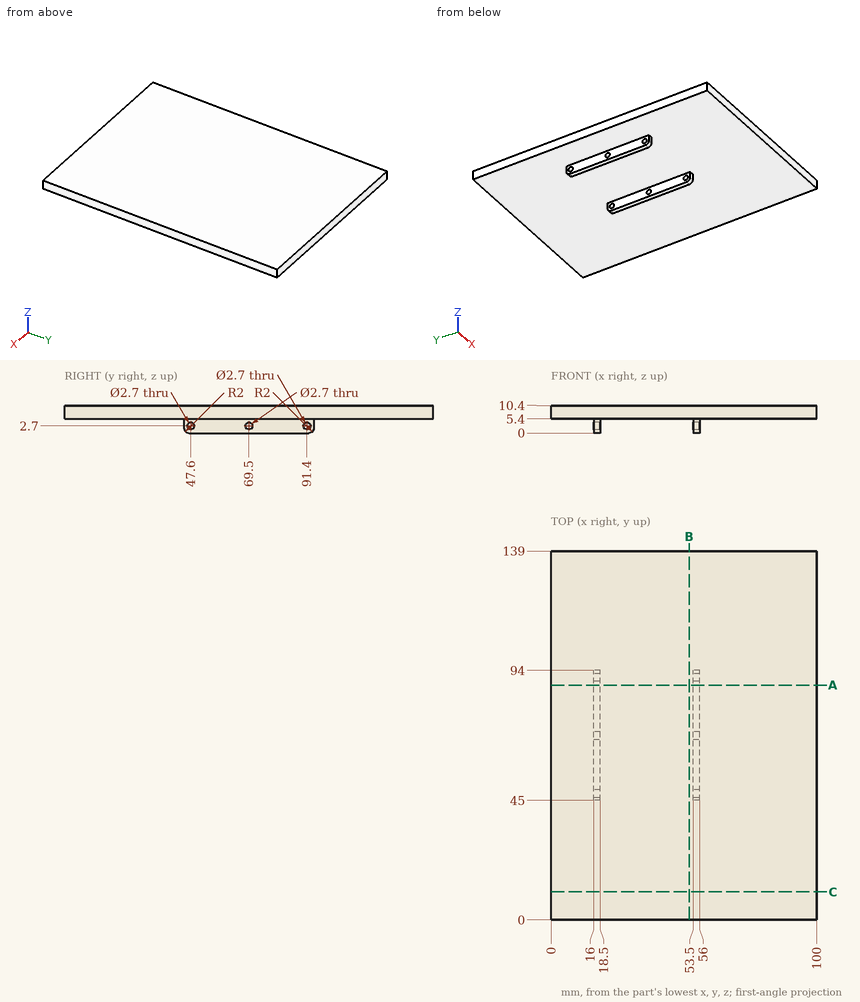
Geometry check sheet. Reference: drawing and pictorial views, mm from the part's lowest x, y, z. Give positions to 0.01 mm unless a question says otherwise; leave off trailing zeros. Write each loop counter-clockwise with the first axis right and the second up, starting at its lowest first coordinate (ties: lowest second). Pieces come first, ordered by that corner, then holes.
Item 1: Gauge pin test, flat ends, axial feed: pin 1 (3 mm diameter, centred on x = 17, z = 3.5, fed in from +Y); pin 2 (1.2 mm diameter, centred on x = 17.5, z = 4.5, fed in from -Y); pin 3 (2 mm diameter, centred on y = 69.5, z = 2.7, fed in from +X); pin 4 (3 mm diameter, centred on y = 69.5, z = 2.7, fed in from +X). Record the tip position at first contact, or that the pin passes through.
Item 2: Scan lines: L1, parallel to Z at x = 55.4, y = 69.5; L2, parallel to X at y = 86.5, z = 0.5; L3, parallel to Z at x = 27.5, y = 78. Record each from-to range of solid material in increasing order.
Item 3: Cross-section at C-C (y = 10.5). Enter the section's corners in (x, z).
Item 4: Cross-section at A-A (y = 88.5). Enter the section's corners in (x, z), and give its area (3 significant figures).
Item 5: Cross-section at B-B (x = 52). Enter the section's corners in (y, z).
Report:
1. pin 1: stops at y = 94
1. pin 2: stops at y = 45
1. pin 3: passes through
1. pin 4: stops at x = 56
2. L1: z = 0 to 1.35, 4.05 to 10.4
2. L2: x = 16 to 18.5, 53.5 to 56
2. L3: z = 5.4 to 10.4
3. outline: (0, 5.4) - (100, 5.4) - (100, 10.4) - (0, 10.4) - close
4. outline: (0, 5.4) - (16, 5.4) - (16, 0) - (18.5, 0) - (18.5, 5.4) - (53.5, 5.4) - (53.5, 0) - (56, 0) - (56, 5.4) - (100, 5.4) - (100, 10.4) - (0, 10.4) - close
4. area: 527 mm2
5. outline: (0, 5.4) - (139, 5.4) - (139, 10.4) - (0, 10.4) - close
